Input: dimensioned drawing with shaded views. Units: mm. Origin: part minimum x, y, z. A direction names the side the tool comes from. Coordinates: 2 decimals unless noted, no trailing zeros. Order: outer loops, then holes, each group sorted by start corner. A loop starts at its lowest first (then second) coordinate and runs counter-clockwise, first axis right, second up.
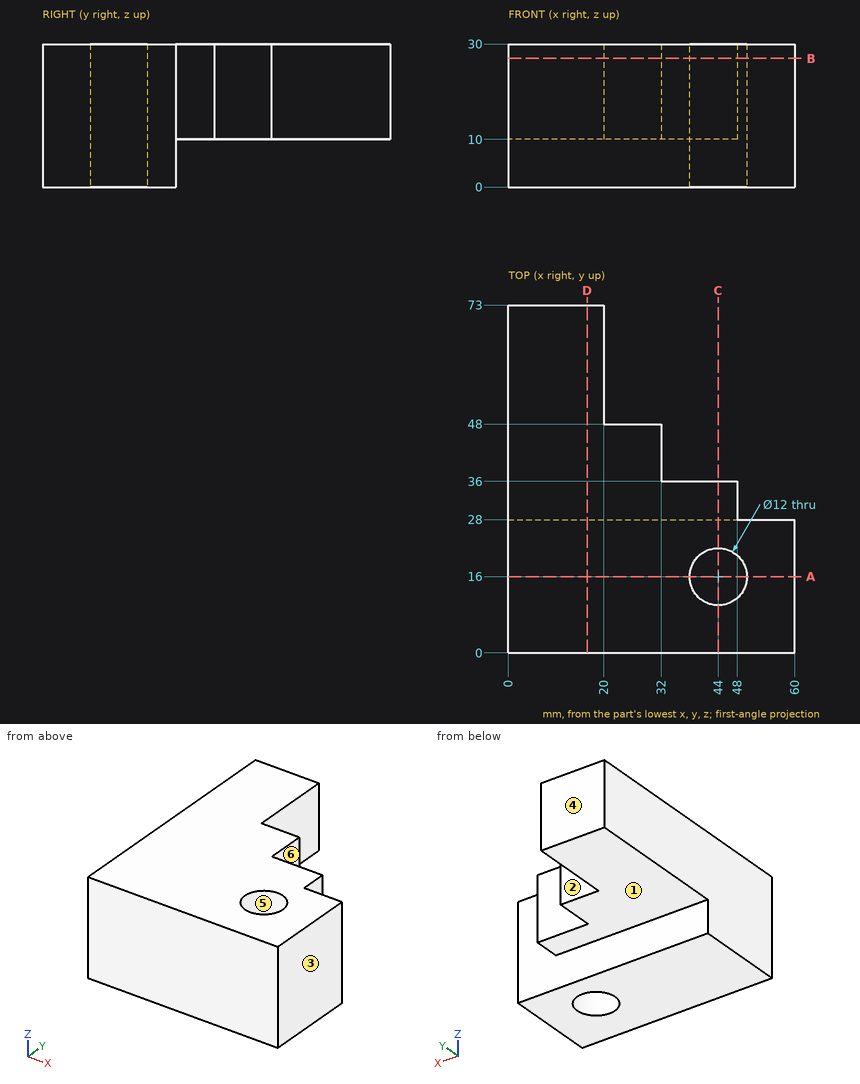
1. Draft query along X for the marked faces 4, 5 and 6. Return one class per face: +X half, -X half, draft (parallel to the pull), parting line (faces both ways), or undercut.
2. Material intervals for line 1 along Y through (x, z) = (44, 14.75); line 2 along X through (y, z) = (50, 12.5); line 3 along Z through (x, y) = (9, 35.5), sorted ascending.
3. Access query for the marked faces 1, 2 and 3. Directions: +Z, -Z, +X, -X, +Y, -Y. A direction counts if a zero-diameter tool reaches every point of the face in a straight line with its end or side. Return the directions, or none.
4. Section query A-A, the plane y = 16. Output: boundary loops of the cut face in (x, z), plus the area to 3 significant figures.
5. Section query D-D, the plane x = 16.5. Output: boundary loops of the cut face in (y, z), plus the area to 3 significant figures.
6. Section query B-B, the plane z = 27. Output: boundary loops of the cut face in (x, y).
7. Section query C-C, the plane x = 44. Output: boundary loops of the cut face in (y, z), plus the area to 3 significant figures.
8. Contact query for flat-ended pins moving along their axis: P1, Ø6, axis at y = 47, z = 15.5, coming from the +X side; P2, Ø3.5, axis at x = 27, z = 16.5, coming from the +Y side; P3, Ø2, axis at x = 40.5, z = 4.5, coming from the +Y side. Output: stop coordinate, or through.
Answer key:
1. face 4: draft
1. face 5: undercut
1. face 6: +X half
2. line 1: y = 0 to 10, 22 to 36
2. line 2: x = 0 to 20
2. line 3: z = 10 to 30
3. face 1: -Z, +X, -X, +Y
3. face 2: +Z, -Z, +X, +Y
3. face 3: +Z, -Z, +X, +Y, -Y
4. outline: (0, 0) - (38, 0) - (38, 30) - (0, 30) - close; (50, 0) - (60, 0) - (60, 30) - (50, 30) - close
4. area: 1,440 mm2
5. outline: (0, 0) - (28, 0) - (28, 10) - (73, 10) - (73, 30) - (0, 30) - close
5. area: 1,740 mm2
6. outline: (0, 0) - (60, 0) - (60, 28) - (48, 28) - (48, 36) - (32, 36) - (32, 48) - (20, 48) - (20, 73) - (0, 73) - close; hole circle Ø12 at (44, 16)
7. outline: (0, 0) - (10, 0) - (10, 30) - (0, 30) - close; (22, 0) - (28, 0) - (28, 10) - (36, 10) - (36, 30) - (22, 30) - close
7. area: 640 mm2
8. P1: stops at x = 32
8. P2: stops at y = 48
8. P3: stops at y = 28
